Part model, mm, in its own coordinate system. A direction names the side the tool comes from. Round coordinates to 2 decimals unless told otherwise and drop trailing zeros. Loops run counter-clockwise (first coordinate to the right, second up) from the corner with the lowest first, then second, coordinate; pieces in that order, holes last. Notation, with made-up numbers: M 53,-6 L 91,-6 A11 cw 91,-1 Z; hole C -5,-24 d9. An arc over 180 degrees is marked long. Put each result on its own line as item: value. Start each with the question number.
1) Slice it at D-D on z = 15.5. Give the cut face in (x, y), then the cut area to 3 significant figures.
2) Slice it at C-C on y = -11. Give the cut face in (x, z).
3) Probe line 1 along Z through (x, y) = (1, -23); line 2 along X through (y, z) = (-28.5, 24); line 3 along Y through (x, z) = (-25.95, -36.83). List the from-to ranges inside material, lowest first.
4) Drop flat-ended pins along their axis: pin 1 Ø1.3 at (x, z) = (26, 34.5) entering from -Y; pin 2 Ø8 at (x, y) = (16, -33.5) entering from +Z; pin 3 Ø6 at (x, y) = (1, -17.5) entering from -Z. Give the stop position or say it passes through.
5) Slice it at B-B on z = 36.83. Give the cut face in (x, y).
6) Slice it at A-A on y = -3.81. State how many separate pieces and enclosed holes the cut face has, then the cut area to 3 significant figures.
7) Pull direction Z, two halves, no side cores. Call faces 1 (the flat face through (-25.273, -3.8, -39.2)), 2 (the flat face through (-27, -4, 41.91)), 3 (the flat face through (25.273, -24, 0)): +Z half, -Z half, draft (parallel to the pull), parting line (faces both ways), or undercut.
8) Which spindle directions (+Z, -Z, +X, -X, +Y, -Y) get a long thin tool onto all of the face, cutting with end or side? Do faces 4 (the flat face through (25.273, -3.8, -39.2)), 5 (the flat face through (-27, -7.62, -37)), 6 (the flat face through (25.273, -3.8, 39.2)), 7 (the flat face through (0, -48.26, 0)). Say none if no direction does.
```python
from build123d import *

# Parameters (mm, degrees)
SKETCH1_W               = 55.626
SKETCH1_H               = 63.5
BOSS_EXTRUDE1_DEPTH     = 50.8
SKETCH2_W               = 50.546
SKETCH2_H               = 58.42
CUT_EXTRUDE1_DEPTH      = 48.26
SKETCH3_W               = 10.16
SKETCH3_H               = 7.62
SKETCH3_R               = 2.159
BOSS_EXTRUDE2_DEPTH     = 2.54
MIRROR2_COPY_1_SKETCH_W = 10.16
MIRROR2_COPY_1_SKETCH_H = 7.62
MIRROR2_COPY_1_SKETCH_R = 2.159
MIRROR2_COPY_1_DEPTH    = 2.54


with BuildPart() as part:
    # Sketch1 → Boss-Extrude1 (new body)
    with BuildSketch(Plane(origin=(0, 0, 0), x_dir=(1, 0, 0), z_dir=(0, 1, 0))):
        Rectangle(SKETCH1_W, SKETCH1_H)
    extrude(amount=-BOSS_EXTRUDE1_DEPTH)

    # Sketch2 → Cut-Extrude1 (cut)
    with BuildSketch(Plane(origin=(0, 0, 0), x_dir=(1, 0, 0), z_dir=(0, 1, 0))):
        Rectangle(SKETCH2_W, SKETCH2_H)
    extrude(amount=-CUT_EXTRUDE1_DEPTH, mode=Mode.SUBTRACT)

    # Sketch3 → Boss-Extrude2 (add)
    with BuildSketch(Plane(origin=(27.813, 0, 0), x_dir=(0, 0, -1), z_dir=(1, 0, 0))):
        with Locations((-36.83, -3.81)):
            Rectangle(SKETCH3_W, SKETCH3_H)
        with Locations((-36.83, -3.81)):
            Circle(SKETCH3_R, mode=Mode.SUBTRACT)
    boss_extrude2 = extrude(amount=-BOSS_EXTRUDE2_DEPTH)

    # Mirror1: Boss-Extrude2 across plane
    add(boss_extrude2.mirror(Plane.XY))

    # Mirror2: Boss-Extrude2 across plane
    add(boss_extrude2.mirror(Plane(origin=(0, 0, 0), x_dir=(0, 0, 1), z_dir=(1, 0, 0))))

    # Mirror2 copy 1 sketch → Mirror2 copy 1 (add)
    with BuildSketch(Plane.ZY.offset(27.813)):
        with Locations((-36.83, -3.81)):
            Rectangle(MIRROR2_COPY_1_SKETCH_W, MIRROR2_COPY_1_SKETCH_H)
        with Locations((-36.83, -3.81)):
            Circle(MIRROR2_COPY_1_SKETCH_R, mode=Mode.SUBTRACT)
    extrude(amount=-MIRROR2_COPY_1_DEPTH)


solid = part.part
```
Recorded:
1. outline: M -27.81,-50.8 L 27.81,-50.8 L 27.81,0 L 25.27,0 L 25.27,-48.26 L -25.27,-48.26 L -25.27,0 L -27.81,0 Z
1. area: 386 mm2
2. outline: M -27.81,-31.75 L 27.81,-31.75 L 27.81,31.75 L -27.81,31.75 Z; hole M -25.27,-29.21 L 25.27,-29.21 L 25.27,29.21 L -25.27,29.21 Z
3. line 1: z = -31.75 to -29.21, 29.21 to 31.75
3. line 2: x = -27.81 to -25.27, 25.27 to 27.81
3. line 3: y = -7.62 to -5.97, -1.65 to 0
4. pin 1: stops at y = -7.62
4. pin 2: stops at z = 31.75
4. pin 3: stops at z = -31.75
5. outline: M -27.81,-7.62 L -25.27,-7.62 L -25.27,-5.97 L -27.81,-5.97 Z; M -27.81,-1.65 L -25.27,-1.65 L -25.27,0 L -27.81,0 Z; M 25.27,-7.62 L 27.81,-7.62 L 27.81,-5.97 L 25.27,-5.97 Z; M 25.27,-1.65 L 27.81,-1.65 L 27.81,0 L 25.27,0 Z
6. separate pieces: 5
6. enclosed holes: 1
6. area: 639 mm2
7. face 1: draft
7. face 2: +Z half
7. face 3: undercut
8. face 4: -Z, +Y, -Y
8. face 5: -Z, +X, -X, -Y
8. face 6: +Z, +Y, -Y
8. face 7: +Y
